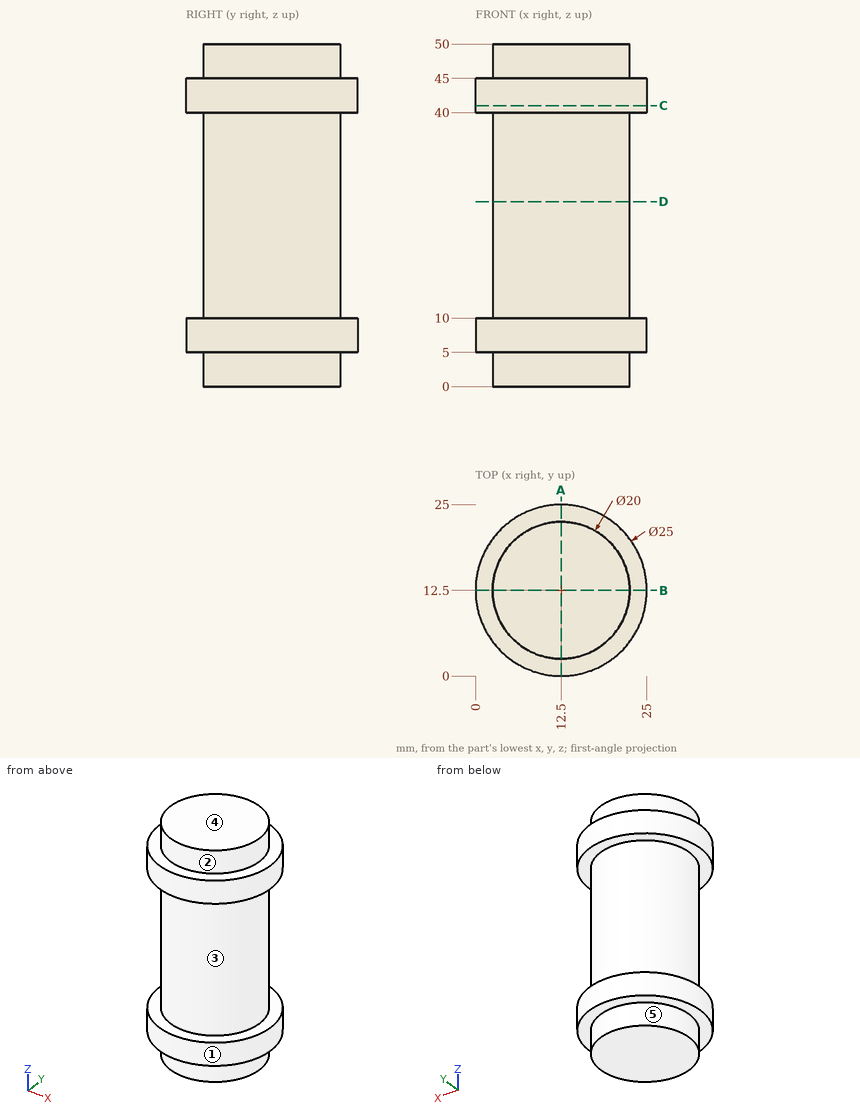
Design review of the part shown in the three views and the two pictorial views. Dimensions are in mm from the part's minimum x, y and z. A direction names the side the tool comes from. Coordinates: 2 decimals unless noted, no trailing zeros. Write each loop counter-clockwise with the first axis right and the second up, starting at its lowest first coordinate (ties: lowest second). Pieces come first, ordered by that corner, then holes. Notation, with made-up numbers: (83, -11) - (127, -11) arc R19 cw to (127, 0) - close; hole circle Ø10 at (80, -38.75). An arc over 180 degrees is marked (long way). Write item = value, one per line.
(1) Consider section D-D, the plane z = 27. Give the boundary of the cut face in (x, y), then the cut area to 3 significant figures.
Result sheet:
outline = circle Ø20 at (12.5, 12.5)
area = 314 mm^2
(2) Mouldability with a two-part tool opening along Z and no side actions: class the marked faces 3, 4 and 5 as pulls with the +Z half, pulls with the -Z half, needs draft (parallel to the pull), parting line crosses it, or undercut.
Result sheet:
face_3 = undercut
face_4 = pulls with the +Z half
face_5 = needs draft
(3) Machinability: for the marked faces 1 and 2, which of the approach directions +Z, -Z, +X, -X, +Y, -Y give a long, thin tool a straight path to every point of the face, cutting with its end or side? Answer none if there is none.
Result sheet:
face_1 = +Z, -Z
face_2 = +Z
(4) For P1, Ø1.5, axis at y = 21.5, z = 21.5, coming from the +X side; P2, Ø6, axis at y = 6.5, z = 28.5, coming from the -X side; P3, Ø5, axis at x = 3.5, z = 37, coming from the +Y side, all flat-tipped, find the tip position at first contact; note any pin that passes through.
Result sheet:
P1 = 18.15
P2 = 2.96
P3 = 20.1
(5) For line 1 (Z direction, x = 5.25, y = 19.75); line 2 (Y direction, x = 20.25, z = 26.5); line 3 (X direction, y = 14, z = 20.5), list the stretches that pass through material, from the lowest coordinate up. Write a range as [from, to].
Result sheet:
line_1 = [5, 10], [40, 45]
line_2 = [6.18, 18.82]
line_3 = [2.61, 22.39]
(6) Consider section A-A, the plane x = 12.5. Give the boundary of the cut face in (y, z).
Result sheet:
outline = (0, 5) - (2.5, 5) - (2.5, 0) - (22.5, 0) - (22.5, 5) - (25, 5) - (25, 10) - (22.5, 10) - (22.5, 40) - (25, 40) - (25, 45) - (22.5, 45) - (22.5, 50) - (2.5, 50) - (2.5, 45) - (0, 45) - (0, 40) - (2.5, 40) - (2.5, 10) - (0, 10) - close
(7) Consider section C-C, the plane z = 41. Give the boundary of the cut face in (x, y), then the cut area to 3 significant figures.
Result sheet:
outline = circle Ø25 at (12.5, 12.5)
area = 491 mm^2
